```python
from build123d import *

# Parameters (mm, degrees)
F1_DEPTH = 2552.7


with BuildPart() as f1:
    # F0 (on Front) → F1 (new body)
    with BuildSketch(Plane.XZ):
        with BuildLine():
            Line((0, 184.15), (0, 0))
            Line((0, 0), (19.05, 0))
            Line((19.05, 0), (19.05, 19.05))
            Line((19.05, 19.05), (19.05, 152.4))
            ThreePointArc((19.05, 152.4), (12.7, 158.75), (19.05, 165.1))
            Line((19.05, 165.1), (19.05, 177.8))
            ThreePointArc((19.05, 177.8), (17.190128, 182.290128), (12.7, 184.15))
            Line((12.7, 184.15), (0, 184.15))
        make_face()
        with BuildLine():
            Line((19.05, 19.05), (19.05, 0))
            Line((19.05, 0), (38.1, 0))
            ThreePointArc((38.1, 0), (32.520384, 13.470384), (19.05, 19.05))
        make_face()
    extrude(amount=-F1_DEPTH)


solid = f1.part
```
Geometry: final body of the model. Coordinates: model frame, mm. A direction names the side the tool comes from. Coordinates: 2 decimals unless noted, no trailing zeros. Loops run counter-clockwise (first coordinate to the right, second up) from the corner with the lowest first, then second, coordinate; pieces in that order, holes last. Notation, with made-up numbers: M 18,6.25 L 69,6.25 A15 cw 69,18.25 Z; hole C -35,70.5 d1. An arc over 180 degrees is marked long. Put each result on its own line as item: value.
(1) Cut plane A-A on y = 246. Return the cut outline in (x, z).
Answer sheet:
outline: M 0,0 L 38.1,0 A19.05 ccw 19.05,19.05 L 19.05,152.4 A6.35 cw 19.05,165.1 L 19.05,177.8 A6.35 ccw 12.7,184.15 L 0,184.15 Z
(2) Cut plane C-C on x = 32. Return the cut outline in (y, z).
Answer sheet:
outline: M 0,0 L 2552.7,0 L 2552.7,13.97 L 0,13.97 Z
(3) First-contact query: pin 1 (1 mm diameter, centred on x = 7.5, y = 1077.5, fed in from -Z); pin 2 (10 mm diameter, centred on y = 818.5, z = 171, fed in from +X). Flat tips, straight axial feed; report the tip coordinate or a pass-through.
Answer sheet:
pin 1: stops at z = 0
pin 2: stops at x = 19.05
(4) Access query for faces 1 (the face through (19.05, 1258, 85)), 2 (the face through (0, 1258, 93)). Directions: +Z, -Z, +X, -X, +Y, -Y. A direction counts if a zero-diameter tool reaches every point of the face in a straight line with its end or side. Return the directions, or none.
Answer sheet:
face 1: +Z, +X, +Y, -Y
face 2: +Z, -Z, -X, +Y, -Y
(5) Material intervals for probe 1 along X at (y, z) = (182, 39); probe 2 along Z at (x, y) = (20, 1236); probe 3 along X at (y, z) = (1565, 161), sorted ascending.
Answer sheet:
probe 1: x = 0 to 19.05
probe 2: z = 0 to 19.03
probe 3: x = 0 to 13.11
(6) Cut plane B-B on z = 57.5. Return the cut outline in (x, y), then the cut area to 3 significant figures.
Answer sheet:
outline: M 0,0 L 19.05,0 L 19.05,2552.7 L 0,2552.7 Z
area: 48,600 mm^2
